The model under review builds one solid part; all positions refer to its coordinate system, in mm. Give positions to 0.01 mm unless a question says otherwise; leave off trailing zeros. Write each loop counter-clockwise with the first axis right and the second up, starting at its lowest first coordinate (ties: lowest second). Pieces come first, ordered by that corner, then holes.
from build123d import *

# Parameters (mm, degrees)
F0_W     = 23.8125
F0_H     = 7.9375
F0_R     = 1.35255
F1_DEPTH = 11.189043
F2_R     = 1.7272
F3_DEPTH = 7.9375


with BuildPart() as f1:
    # F0 (on Top) → F1 (new body)
    with BuildSketch(Plane.XY):
        with Locations((11.90625, 3.96875)):
            Rectangle(F0_W, F0_H)
        with Locations((3.96875, 3.96875)):
            Circle(F0_R, mode=Mode.SUBTRACT)
        with Locations((19.84375, 3.96875)):
            Circle(F0_R, mode=Mode.SUBTRACT)
    extrude(amount=F1_DEPTH)

    # F2 (on face) → F3 (cut, through all)
    with BuildSketch(Plane.XZ):
        with Locations((11.90625, 7.220293)):
            Circle(F2_R)
    extrude(amount=-F3_DEPTH, mode=Mode.SUBTRACT)


solid = f1.part
1) Consider section C-C, the plane x = 3.75. Give the boundary of the cut face in (y, z), then the cut area to 3 significant figures.
2) Consider section A-A, the plane z = 8.5. Give the boundary of the cut face in (x, y), then the cut area to 3 significant figures.
3) Consider section D-D, the plane y = 6.5. Give the boundary of the cut face in (x, z).
4) The part is to be moulded in two halves that separate along Y. For faces 1 (the cylindrical face through (19.55, 2.65, 5.52)), 2 (the flat face through (23.812, 4, 6)), 3 (the flat face through (12, 7.938, 4)), say which applies: +Y half, -Y half, draft (parallel to the pull), parting line (faces both ways), or undercut.
5) To check wall thickness, follow probe 1 along X at (y, z) = (3.5, 10.5); probe 2 along X at (y, z) = (4.5, 6.75); probe 3 along Y at (x, z) = (20.5, 4.5). State the ranges of each line that lie inside material, in increasing order.
6) Insertion check: pin 1 (3 mm diameter, centred on x = 18, z = 6, fed in from -Y). The pin has a flat end and moves straight along its axis. Give the tip position at first contact, or say it passes through.
7) Consider section B-B, the plane y = 3.5. Give the boundary of the cut face in (x, z), then the cut area to 3 significant figures.
Answer block:
1. outline: (0, 0) - (2.63, 0) - (2.63, 11.19) - (0, 11.19) - close; (5.3, 0) - (7.94, 0) - (7.94, 11.19) - (5.3, 11.19) - close
1. area: 58.9 mm2
2. outline: (0, 0) - (10.75, 0) - (10.75, 7.94) - (0, 7.94) - close; (13.07, 0) - (23.81, 0) - (23.81, 7.94) - (13.07, 7.94) - close; hole circle Ø2.71 at (3.97, 3.97); hole circle Ø2.71 at (19.84, 3.97)
2. area: 159 mm2
3. outline: (0, 0) - (23.81, 0) - (23.81, 11.19) - (0, 11.19) - close; hole circle Ø3.45 at (11.91, 7.22)
4. face 1: undercut
4. face 2: draft
4. face 3: +Y half
5. probe 1: x = 0 to 2.7, 5.24 to 18.58, 21.11 to 23.81
5. probe 2: x = 0 to 2.72, 5.21 to 10.24, 13.57 to 18.6, 21.09 to 23.81
5. probe 3: y = 0 to 2.79, 5.15 to 7.94
6. pin 1: stops at y = 0
7. outline: (0, 0) - (2.7, 0) - (2.7, 11.19) - (0, 11.19) - close; (5.24, 0) - (18.58, 0) - (18.58, 11.19) - (5.24, 11.19) - close; (21.11, 0) - (23.81, 0) - (23.81, 11.19) - (21.11, 11.19) - close; hole circle Ø3.45 at (11.91, 7.22)
7. area: 200 mm2
